```python
from build123d import *

# Parameters (mm, degrees)
SKETCH_1_R          = 6.5
EXTRUDE_1_DEPTH     = 8
SKETCH_2_R          = 2
EXTRUDE_2_DEPTH     = 46
SKETCH_6_R          = 5.5
SKETCH_6_R_2        = 3.5
CUT_EXTRUDE_1_DEPTH = 2
CUT_EXTRUDE_START   = -2
SKETCH_7_R          = 5.5
SKETCH_7_R_2        = 3.5
CUT_EXTRUDE_2_DEPTH = 2
FILLET_2_R          = 0.5


with BuildPart() as part:
    # 草图1 → 凸台-拉伸1 (new body)
    with BuildSketch(Plane(origin=(0, 0, 0), x_dir=(1, 0, 0), z_dir=(0, 1, 0))):
        with Locations(Location((0, 0, 0), (0, 0, 270))):
            Circle(SKETCH_1_R)
    extrude(amount=EXTRUDE_1_DEPTH)

    # 草图2 → 凸台-拉伸2 (add)
    with BuildSketch(Plane(origin=(0, 8, 0), x_dir=(1, 0, 0), z_dir=(0, 1, 0))):
        with Locations(Location((0, 0, 0), (0, 0, 270))):
            Circle(SKETCH_2_R)
    extrude(amount=EXTRUDE_2_DEPTH)

    # 草图4 → 旋转1 (revolve)
    with BuildSketch(Plane.XY):
        with BuildLine():
            Line((0, 54), (0, 56))
            Line((0, 56), (0, 56.8))
            Line((0, 56.8), (1.95, 56.8))
            Line((1.95, 56.8), (1.95, 55.555590279))
            ThreePointArc((1.95, 55.555590279), (1.780042303, 55.088161527), (1.5, 54.677124344))
            Line((1.5, 54.677124344), (1.5, 54))
            Line((1.5, 54), (0, 54))
        make_face()
    revolve(axis=Axis((0, 54, 0), (0, 1, 0)))

    # 草图5 → 切除-旋转1 (revolve, cut)
    with BuildSketch(Plane.XY, mode=Mode.PRIVATE) as cut_revolve_1_sk:
        Polygon((-6.5, 8), (-6.5, 5), (-6.5, 3), (-6.5, 0), (-6, 3), (-6, 5), align=None)
    revolve(cut_revolve_1_sk.sketch.rotate(Axis((0, 0, 0), (0, 1, 0)), 270), axis=Axis((0, 0, 0), (0, 1, 0)), mode=Mode.SUBTRACT)

    # 草图6 → 切除-拉伸1 (cut)
    with BuildSketch(Plane.XZ):
        with Locations(Location((0, 0, 0), (0, 0, 270))):
            Circle(SKETCH_6_R)
        with Locations(Location((0, 0, 0), (0, 0, 270))):
            Circle(SKETCH_6_R_2, mode=Mode.SUBTRACT)
    extrude(amount=-CUT_EXTRUDE_1_DEPTH, mode=Mode.SUBTRACT)

    # 草图7 → 切除-拉伸2 (cut)
    with BuildSketch(Plane(origin=(0, 8, 0), x_dir=(1, 0, 0), z_dir=(0, 1, 0)).offset(CUT_EXTRUDE_START)):
        with Locations(Location((0, 0, 0), (0, 0, 90))):
            Circle(SKETCH_7_R)
        with Locations(Location((0, 0, 0), (0, 0, 90))):
            Circle(SKETCH_7_R_2, mode=Mode.SUBTRACT)
    extrude(amount=CUT_EXTRUDE_2_DEPTH, mode=Mode.SUBTRACT)

    # 圆角2
    fillet_2_edges = [part.edges().sort_by_distance(p)[0] for p in [
        (0, 0, 3.5),
        (0, 8, 3.5),
    ]]
    fillet(fillet_2_edges, radius=FILLET_2_R)


solid = part.part
```
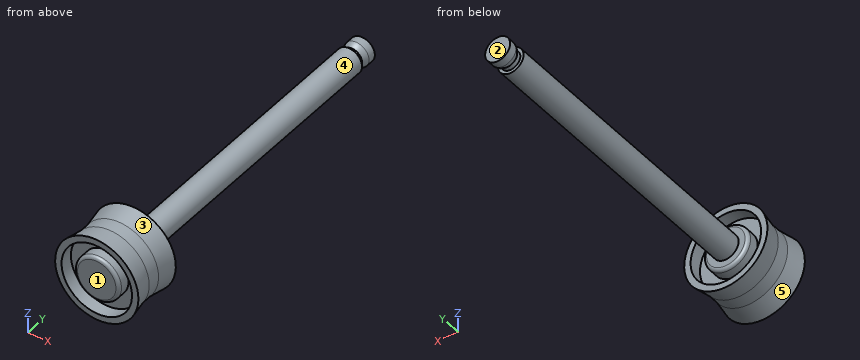
Can you work these out from the model? Positions are in its coordinate system, mm. Face numbers are marked on the shaded views. A direction names the side the tool comes from. Give positions to 0.01 mm unless a question says otherwise; leave off trailing zeros. Loops run counter-clockwise (first coordinate to the right, second up) from the corner with the lowest first, then second, coordinate; pieces in that order, holes last. Notation, with made-up numbers: M 40.25,-18 L 69.25,-18 A23 ccw 69.25,-8 Z; hole C 40.25,67.5 d5. An arc over 180 degrees is marked long. Use one line per item in the form item = value. Start each with the question number.
(1) I'm going to push flat-ended pins straight in: P1, Ø1, axis at x = -4, y = 27.5, coming from the +Z side; P2, Ø1, axis at y = 45.5, z = -1, coming from the -X side; P3, Ø4, axis at y = 31, z = 0, coming from the -X side; P4, Ø6.5, axis at x = 1.5, z = -1.5, coming from the +Y side. Where does each tip first touch, or does it pass through?
(2) I want a section at A-A, the plane y = 44. Write out the boundary of the cut face in (x, z), and give its area (3 significant figures).
(3) Please list where these lines run through material, in increasing order: line 1 (X direction, y = 1.45, z = 0); line 2 (Y direction, x = 4.75, z = -1.75); line 3 (X direction, y = 7.4, z = 0).
(4) On a 3-axis mill with a long thin cutter (end or side, diameter ignored), from which of +Z, -Z, +X, -X, +Y, -Y can I reach the whole of each face in a straight line? I mean the marked faces 4 and 5. Say none if no direction works.
(5) Thinking about a two-plate mould opening in Y: for the marked faces 1, 2 and 3, which applies, released by +Y, released by -Y, zero draft, split by the parting line, or undercut?
Worked out:
q1.P1 = through
q1.P2 = -1.94
q1.P3 = -2
q1.P4 = 56.8
q2.outline = C 0,0 d4
q2.area = 12.6 mm²
q3.line_1 = -6.26 to -5.5, -3.5 to 3.5, 5.5 to 6.26
q3.line_2 = 2 to 6
q3.line_3 = -6.4 to -5.5, -3.5 to 3.5, 5.5 to 6.4
q4.face_4 = +Y
q4.face_5 = none
q5.face_1 = released by -Y
q5.face_2 = released by +Y
q5.face_3 = undercut
